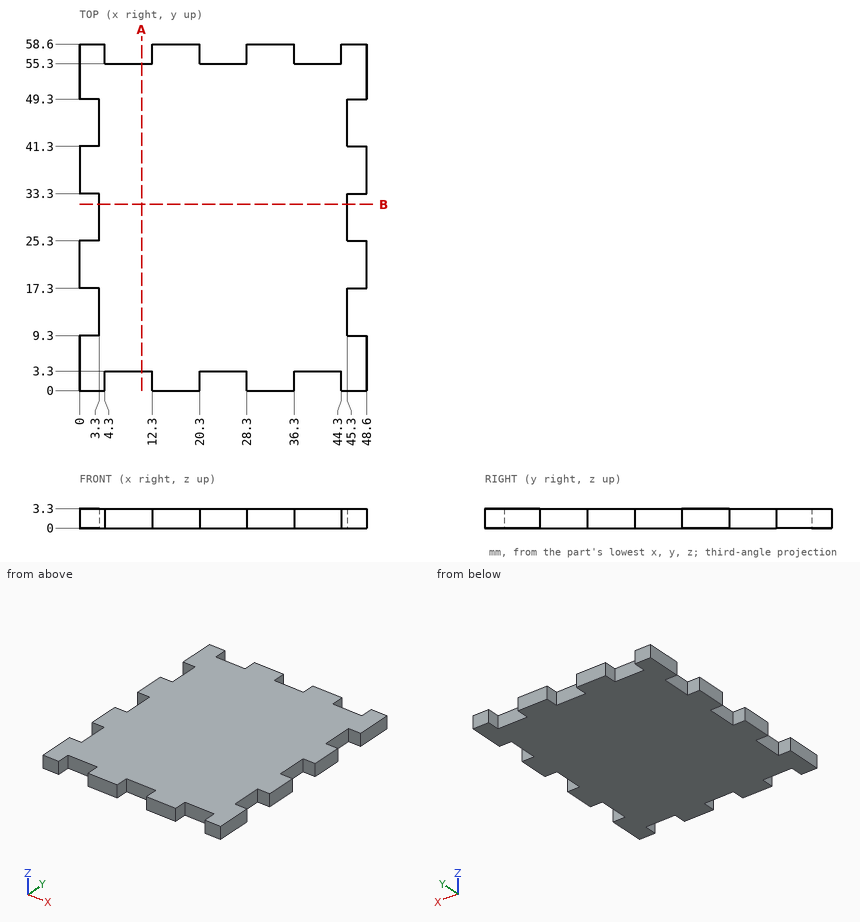
Check sheet for the drawn part. Datum: minimum x, y, z corner. Units: mm. Round coordinates to 2 decimals unless told otherwise and drop trailing zeros. Order: outer loops, then holes, each group sorted by start corner. A loop starts at its lowest first (then second) coordinate and runs counter-clockwise, first axis right, second up.
1) Go/stop test with flat-tipped pins: pin 1 Ø1 at (x, z) = (22.5, 1.5) entering from +Y; pin 2 Ø1 at (y, z) = (46, 1) entering from +X; pin 3 Ø1 at (y, z) = (46.5, 1) entering from -X. Record where each tip stops, or that it passes through.
2) Scan lines: line 1 (X direction, y = 56, z = 2.45); line 2 (X direction, y = 45, z = 1.3); line 3 (Y direction, x = 26, z = 1.65). Record each from-to range of solid material in increasing order.
3) Section check A-A (x = 10.5). Record the boundary of the cut face in (y, z).
4) Section check B-B (y = 31.5). Record the boundary of the cut face in (x, z).
Result:
1. pin 1: stops at y = 55.3
1. pin 2: stops at x = 45.3
1. pin 3: stops at x = 3.3
2. line 1: x = 0 to 4.3, 12.3 to 20.3, 28.3 to 36.3, 44.3 to 48.6
2. line 2: x = 3.3 to 45.3
2. line 3: y = 3.3 to 55.3
3. outline: (3.3, 0) - (55.3, 0) - (55.3, 3.3) - (3.3, 3.3) - close
4. outline: (3.3, 0) - (45.3, 0) - (45.3, 3.3) - (3.3, 3.3) - close
